Here's how the part is built. I have some questions about the finished solid (model axes, mm). Face numbers are marked on the shaded views. A direction names the side the tool comes from. Coordinates: 2 decimals unless noted, no trailing zeros. Write each loop counter-clockwise with the first axis right and the second up, starting at its lowest first coordinate (ties: lowest second). Pieces come first, ordered by that corner, then holes.
```python
from build123d import *

# Parameters (mm, degrees)
SKETCH1_W               = 113
SKETCH1_H               = 54
BOSS_EXTRUDE1_DEPTH     = 10
SKETCH1_3_W             = 113
SKETCH1_3_H             = 54
SKETCH1_3_R             = 1.5
BOSS_EXTRUDE2_DEPTH     = 5.4
BOSS_EXTRUDE5_START     = 5.4
SKETCH1_4_W             = 113
SKETCH1_4_H             = 54
SKETCH1_4_R             = 3.75
SKETCH1_4_R_2           = 4.5
SKETCH1_4_W_2           = 51.62
SKETCH1_4_H_2           = 39.38
BOSS_EXTRUDE5_DEPTH     = 6
CUT_EXTRUDE_THIN1_START = 5.4
CUT_EXTRUDE_THIN1_DEPTH = 6
CUT_EXTRUDE1_DEPTH      = 5
FILLET1_R               = 1.5
CUT_EXTRUDE2_DEPTH      = 0.2
CHAMFER1_SIZE           = 3
CHAMFER1_SIZE2          = 5.196152423
SKETCH4_W               = 26.49
SKETCH4_H               = 4
CUT_EXTRUDE3_DEPTH      = 5
SKETCH5_W               = 14
SKETCH5_H               = 8.4
CUT_EXTRUDE4_DEPTH      = 5
BOSS_EXTRUDE6_DEPTH     = 25.4
SKETCH7_R               = 3.25
CUT_EXTRUDE5_DEPTH      = 46.907223847
CUT_EXTRUDE8_START      = -3
SKETCH7_4_R             = 8.5
SKETCH7_4_R_2           = 3.25
CUT_EXTRUDE8_DEPTH      = 43.907223847
SKETCH8_R               = 3.25
CUT_EXTRUDE6_DEPTH      = 60.675369484
CUT_EXTRUDE9_START      = -3
SKETCH8_5_R             = 8.5
SKETCH8_5_R_2           = 3.25
CUT_EXTRUDE9_DEPTH      = 25.4
BOSS_EXTRUDE9_REACH     = 89.6


with BuildPart() as part:
    # Sketch1 → Boss-Extrude1 (new body)
    with BuildSketch(Plane(origin=(0, 0, 0), x_dir=(1, 0, 0), z_dir=(0, 1, 0))):
        Rectangle(SKETCH1_W, SKETCH1_H)
        Polygon((-53.5, -16.07179677), (-53.5, 16.07179677), (-53.5, 24), (-45.57179677, 24), (45.57179677, 24), (53.5, 24), (53.5, 16.07179677), (53.5, -16.07179677), (53.5, -24), (45.57179677, -24), (-45.57179677, -24), (-53.5, -24), align=None, mode=Mode.SUBTRACT)
    extrude(amount=-BOSS_EXTRUDE1_DEPTH)

    # Sketch1<3> → Boss-Extrude2 (add)
    with BuildSketch(Plane(origin=(0, 0, 0), x_dir=(1, 0, 0), z_dir=(0, 1, 0))):
        Rectangle(SKETCH1_3_W, SKETCH1_3_H)
        Polygon((-53.5, -16.07179677), (-53.5, 16.07179677), (-53.5, 24), (-45.57179677, 24), (45.57179677, 24), (53.5, 24), (53.5, 16.07179677), (53.5, -16.07179677), (53.5, -24), (45.57179677, -24), (-45.57179677, -24), (-53.5, -24), align=None, mode=Mode.SUBTRACT)
        with BuildLine():
            Line((-53.5, 24), (-53.5, 16.07179677))
            ThreePointArc((-53.5, 16.07179677), (-47.550252532, 18.050252532), (-45.57179677, 24))
            Line((-45.57179677, 24), (-53.5, 24))
        make_face()
        with Locations((-50.4, 20.575)):
            Circle(SKETCH1_3_R, mode=Mode.SUBTRACT)
        with BuildLine():
            ThreePointArc((-45.57179677, -24), (-47.550252532, -18.050252532), (-53.5, -16.07179677))
            Line((-53.5, -16.07179677), (-53.5, -24))
            Line((-53.5, -24), (-45.57179677, -24))
        make_face()
        with Locations((-50.4, -20.575)):
            Circle(SKETCH1_3_R, mode=Mode.SUBTRACT)
        with BuildLine():
            Line((53.5, 24), (45.57179677, 24))
            ThreePointArc((45.57179677, 24), (47.550252532, 18.050252532), (53.5, 16.07179677))
            Line((53.5, 16.07179677), (53.5, 24))
        make_face()
        with Locations((50.4, 20.575)):
            Circle(SKETCH1_3_R, mode=Mode.SUBTRACT)
        with BuildLine():
            ThreePointArc((53.5, -16.07179677), (47.550252532, -18.050252532), (45.57179677, -24))
            Line((45.57179677, -24), (53.5, -24))
            Line((53.5, -24), (53.5, -16.07179677))
        make_face()
        with Locations((50.4, -20.575)):
            Circle(SKETCH1_3_R, mode=Mode.SUBTRACT)
    extrude(amount=BOSS_EXTRUDE2_DEPTH)

    # Sketch1<4> → Boss-Extrude5 (add)
    with BuildSketch(Plane(origin=(0, 0, 0), x_dir=(1, 0, 0), z_dir=(0, 1, 0)).offset(BOSS_EXTRUDE5_START)):
        Rectangle(SKETCH1_4_W, SKETCH1_4_H)
        with Locations((42.78, -3.495)):
            Circle(SKETCH1_4_R, mode=Mode.SUBTRACT)
        with Locations((44.69, 12.41)):
            Circle(SKETCH1_4_R_2, mode=Mode.SUBTRACT)
        with Locations((2.01, 0.81)):
            Rectangle(SKETCH1_4_W_2, SKETCH1_4_H_2, mode=Mode.SUBTRACT)
    extrude(amount=BOSS_EXTRUDE5_DEPTH)

    # Sketch1<5> → Cut-Extrude-Thin1 (cut)
    with BuildSketch(Plane(origin=(0, 0, 0), x_dir=(1, 0, 0), z_dir=(0, 1, 0)).offset(CUT_EXTRUDE_THIN1_START)):
        Polygon((49.424523111, -13.683696801), (44.828329033, -18.279890879), (44.828329033, -22.537250192), (32.828329033, -22.537250192), (32.828329033, -14.037250192), (40.585688346, -14.037250192), (45.181882424, -9.441056114), (44.722263016, -8.981436706), (40.316449531, -13.387250192), (32.178329033, -13.387250192), (32.178329033, -23.187250192), (45.478329033, -23.187250192), (45.478329033, -18.549129694), (49.884142519, -14.143316209), align=None)
    extrude(amount=CUT_EXTRUDE_THIN1_DEPTH, mode=Mode.SUBTRACT)

    # Sketch2 → Cut-Extrude1 (cut)
    with BuildSketch(Plane.XZ.offset(-5.4)):
        Polygon((32.828329033, 14.037250192), (32.828329033, 22.537250192), (44.828329033, 22.537250192), (44.828329033, 18.279890879), (49.424523111, 13.683696801), (45.181882424, 9.441056114), (40.585688346, 14.037250192), align=None)
    extrude(amount=-CUT_EXTRUDE1_DEPTH, mode=Mode.SUBTRACT)

    # Fillet1
    fillet1_edges = [part.edges().sort_by_distance(p)[0] for p in [
        (44.828329033, 10.9, 18.279890879),
        (44.828329033, 10.9, 22.537250192),
        (32.828329033, 10.9, 22.537250192),
        (32.828329033, 10.9, 14.037250192),
        (40.585688346, 10.9, 14.037250192),
        (40.316449531, 8.4, 13.387250192),
        (32.178329033, 8.4, 13.387250192),
        (32.178329033, 8.4, 23.187250192),
        (45.478329033, 8.4, 23.187250192),
        (45.478329033, 8.4, 18.549129694),
    ]]
    fillet(fillet1_edges, radius=FILLET1_R)

    # Sketch3 → Cut-Extrude2 (cut)
    with BuildSketch(Plane(origin=(0, 11.4, 0), x_dir=(1, 0, 0), z_dir=(0, 1, 0))):
        Polygon((37.138989205, -15.537250192), (38.828329033, -17.22659002), (40.517668861, -15.537250192), (41.578329033, -16.597910363), (39.888989205, -18.287250192), (41.578329033, -19.97659002), (40.517668861, -21.037250192), (38.828329033, -19.347910363), (37.138989205, -21.037250192), (36.078329033, -19.97659002), (37.767668861, -18.287250192), (36.078329033, -16.597910363), align=None)
    extrude(amount=-CUT_EXTRUDE2_DEPTH, mode=Mode.SUBTRACT)

    # Chamfer1
    chamfer1_edges = [part.edges().sort_by_distance(p)[0] for p in [
        (-23.8, 11.4, -0.81),
        (2.01, 11.4, 18.88),
        (27.82, 11.4, -0.81),
        (2.01, 11.4, -20.5),
    ]]
    chamfer1_side = [part.faces().sort_by_distance(p)[0] for p in [
        (0, 11.4, -25.7476023),
    ]]
    chamfer(chamfer1_edges, length=CHAMFER1_SIZE, length2=CHAMFER1_SIZE2, reference=chamfer1_side[0])

    # Sketch4 → Cut-Extrude3 (cut)
    with BuildSketch(Plane.ZY.offset(56.5)):
        with Locations((1.895, -3.6)):
            Rectangle(SKETCH4_W, SKETCH4_H)
    extrude(amount=-CUT_EXTRUDE3_DEPTH, mode=Mode.SUBTRACT)

    # Sketch5 → Cut-Extrude4 (cut)
    with BuildSketch(Plane(origin=(56.5, 0, 0), x_dir=(0, 0, -1), z_dir=(1, 0, 0))):
        with Locations((12.23, -5.8)):
            Rectangle(SKETCH5_W, SKETCH5_H)
    extrude(amount=-CUT_EXTRUDE4_DEPTH, mode=Mode.SUBTRACT)

    # Sketch6 → Boss-Extrude6 (add)
    with BuildSketch(Plane(origin=(56.5, 0, 0), x_dir=(0, 0, -1), z_dir=(1, 0, 0))):
        Polygon((47.806461925, 11.4), (49.527191234, 8.942543867), (28.720729309, -5.626297616), (43.289570792, -26.432759541), (38.066945953, -30.089680823), (24, -10), (27, -10), (27, -3.168841483), (27, 11.4), align=None)
    boss_extrude6 = extrude(amount=-BOSS_EXTRUDE6_DEPTH)

    # Sketch7 → Cut-Extrude5 (cut, through all)
    with BuildSketch(Plane(origin=(0, -17.269631064, -12.092325853), x_dir=(1, 0, 0), z_dir=(0, -0.819152044, -0.573576436))):
        with Locations((43.8, -32.99953239)):
            Circle(SKETCH7_R)
    cut_extrude5 = extrude(amount=-CUT_EXTRUDE5_DEPTH, mode=Mode.SUBTRACT)

    # Sketch7<4> → Cut-Extrude8 (cut, through all)
    with BuildSketch(Plane(origin=(0, -17.269631064, -12.092325853), x_dir=(1, 0, 0), z_dir=(0, -0.819152044, -0.573576436)).offset(CUT_EXTRUDE8_START)):
        with Locations((43.8, -32.99953239)):
            Circle(SKETCH7_4_R)
        with Locations((43.8, -32.99953239)):
            Circle(SKETCH7_4_R_2, mode=Mode.SUBTRACT)
    cut_extrude8 = extrude(amount=-CUT_EXTRUDE8_DEPTH, mode=Mode.SUBTRACT)

    # Sketch8 → Cut-Extrude6 (cut, through all)
    with BuildSketch(Plane(origin=(0, 11.643333448, -16.628403456), x_dir=(-1, 0, 0), z_dir=(0, 0.573576436, -0.819152044))):
        with Locations((-43.8, -33.782326761)):
            Circle(SKETCH8_R)
    cut_extrude6 = extrude(amount=-CUT_EXTRUDE6_DEPTH, mode=Mode.SUBTRACT)

    # Sketch8<5> → Cut-Extrude9 (cut)
    with BuildSketch(Plane(origin=(0, 11.643333448, -16.628403456), x_dir=(-1, 0, 0), z_dir=(0, 0.573576436, -0.819152044)).offset(CUT_EXTRUDE9_START)):
        with Locations((-43.8, -33.782326761)):
            Circle(SKETCH8_5_R)
        with Locations((-43.8, -33.782326761)):
            Circle(SKETCH8_5_R_2, mode=Mode.SUBTRACT)
    cut_extrude9 = extrude(amount=-CUT_EXTRUDE9_DEPTH, mode=Mode.SUBTRACT)

    # Mirror1: Boss-Extrude6, Cut-Extrude5, Cut-Extrude8, Cut-Extrude6, Cut-Extrude9 across plane
    add(boss_extrude6.mirror(Plane(origin=(0, 0, 0), x_dir=(0, 0, 1), z_dir=(1, 0, 0))))
    add(cut_extrude5.mirror(Plane(origin=(0, 0, 0), x_dir=(0, 0, 1), z_dir=(1, 0, 0))), mode=Mode.SUBTRACT)
    add(cut_extrude8.mirror(Plane(origin=(0, 0, 0), x_dir=(0, 0, 1), z_dir=(1, 0, 0))), mode=Mode.SUBTRACT)
    add(cut_extrude6.mirror(Plane(origin=(0, 0, 0), x_dir=(0, 0, 1), z_dir=(1, 0, 0))), mode=Mode.SUBTRACT)
    add(cut_extrude9.mirror(Plane(origin=(0, 0, 0), x_dir=(0, 0, 1), z_dir=(1, 0, 0))), mode=Mode.SUBTRACT)

    # Sketch9 → Boss-Extrude9 (add, up to next)
    with BuildSketch(Plane.ZY.offset(-31.1), mode=Mode.PRIVATE) as boss_extrude9_sk1:
        Polygon((-27, 11.4), (-35.565845727, -0.833295501), (-27, -6.83116525), align=None)
    boss_extrude9_tool1 = extrude(boss_extrude9_sk1.sketch, amount=BOSS_EXTRUDE9_REACH, mode=Mode.PRIVATE) - part.part
    add(boss_extrude9_tool1.solids().sort_by_distance((31.1, 1.24518, -29.855282))[0])


solid = part.part
```
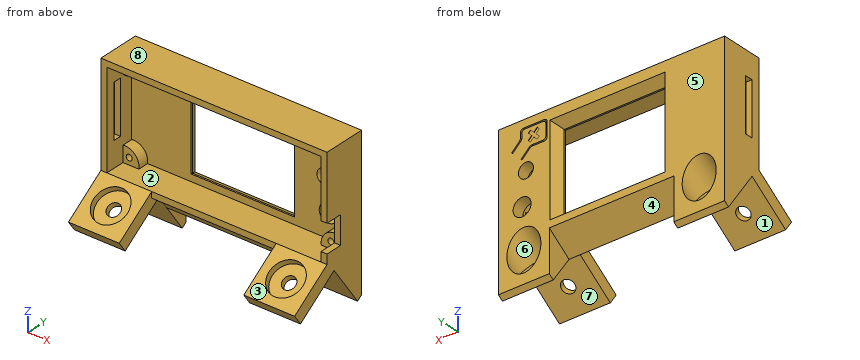
1) Imagine slicing it at D-D on x = -38.5. Please give me the cut outline in (y, z), then the cut area to 3 significant figures.
Values follow:
outline: (-30.09, -38.07) - (-26.43, -43.29) - (-5.63, -28.72) - (8.94, -49.53) - (11.4, -47.81) - (11.4, -40.42) - (7.93, -42.85) - (0.3, -31.96) - (11.4, -24.19) - (11.4, 27) - (-10, 27) - (-10, 24) - (5.4, 24) - (5.4, -24) - (-10, -24) - (-14.24, -26.97) - (-12.31, -29.74) - (-23.19, -37.36) - (-25.13, -34.59) - close
area: 640 mm2
2) I need wall thicknesses on probe 1 along X at (y, z) = (7, -12); probe 2 along X at (y, z) = (3, 5.5); probe 3 along Z at (x, y) = (-50.4, 1.4) (3 decimals). Which ranges of each line are inside material? Lowest first, please.
Values follow:
probe 1: x = -56.5 to -24.26, 28.28 to 40.21, 49.17 to 56.5
probe 2: x = -56.5 to -53.5, 53.5 to 56.5
probe 3: z = -38.755 to -33.525, -32.766 to -22.075, -19.075 to -16.322, 16.322 to 19.075, 22.075 to 27
3) Imagine slicing it at B-B on x = -6. Please give me the cut outline in (y, z).
Values follow:
outline: (-10, -27) - (-6.83, -27) - (-0.83, -35.57) - (11.4, -27) - (11.4, -23.5) - (6.2, -20.5) - (5.4, -20.5) - (5.4, -24) - (-10, -24) - close; (-10, 24) - (5.4, 24) - (5.4, 18.88) - (6.2, 18.88) - (11.4, 21.88) - (11.4, 27) - (-10, 27) - close
4) Will these pins go through, and if not, where does the flat tip stop? pin 1 (0.9 mm diameter, centred on x = 55, y = -6, fed in from -Z); pin 2 (12 mm diameter, centred on x = -38, y = -19, fed in from +Z); pin 3 (12 mm diameter, centred on x = -30, y = -13, fed in from -Z).
Values follow:
pin 1: stops at z = -29.3
pin 2: stops at z = -26.1
pin 3: stops at z = -38.01
5) On a 3-axis mill with a long thin cutter (end or side, diameter ignored), from which of +Z, -Z, +X, -X, +Y, -Y can I reach the whole of each face in a straight line? I mean the marked faces 1, 2, 3, 4 and 5. Say none if no direction works.
Values follow:
face 1: -Z, +X, -X
face 2: -Y
face 3: +Z, +X, -X, -Y
face 4: -Z, +Y
face 5: +Z, -Z, +X, -X, +Y
6) We'd pull the mould along Z, two halves only. Please class the marked faces 6, 7 and 8: pulls with the +Z half, pulls with the -Z half, needs draft (parallel to the pull), parting line crosses it, or undercut.
Values follow:
face 6: undercut
face 7: pulls with the -Z half
face 8: pulls with the +Z half
7) Imagine slicing it at A-A on z = -4. Please give me the cut outline in (x, y).
Values follow:
outline: (-56.5, -10) - (-53.5, -10) - (-53.5, -5.6) - (-56.5, -5.6) - close; (-56.5, -1.6) - (-53.5, -1.6) - (-53.5, 5.4) - (-23.8, 5.4) - (-23.8, 6.2) - (-26.8, 11.4) - (-56.5, 11.4) - close; (27.82, 5.4) - (53.5, 5.4) - (53.5, -10) - (56.5, -10) - (56.5, 11.4) - (30.82, 11.4) - (27.82, 6.2) - close
8) Imagine slicing it at C-C on z = 5. Please give me the cut outline in (x, y).
Values follow:
outline: (-56.5, -10) - (-53.5, -10) - (-53.5, -5.6) - (-56.5, -5.6) - close; (-56.5, -1.6) - (-53.5, -1.6) - (-53.5, 5.4) - (-23.8, 5.4) - (-23.8, 6.2) - (-26.8, 11.4) - (-56.5, 11.4) - close; (27.82, 5.4) - (39.35, 5.4) - (39.35, 11.4) - (30.82, 11.4) - (27.82, 6.2) - close; (46.21, 5.4) - (53.5, 5.4) - (53.5, -10) - (56.5, -10) - (56.5, 11.4) - (46.21, 11.4) - close
